The listing builds one solid part. Answer for the finished solid, in the listing's coordinates (mm). A direction names the side the tool comes from. Round coordinates to 2 decimals unless told otherwise and drop trailing zeros. Write each loop counter-clockwise with the first axis right and the second up, starting at its lowest first coordinate (ties: lowest second). Pieces come first, ordered by that corner, then holes. Notation, with made-up numbers: M -10,19 L 45,19 A12 cw 45,38 Z; hole C 81.5,7.25 d6. An arc over 180 degrees is marked long. Write each question's results on one line, items separated by ' | '.
from build123d import *

# Parameters (mm, degrees)
BOSS_EXTRUDE1_DEPTH     = 38.1
CUT_EXTRUDE1_DEPTH      = 35.56
CUT_EXTRUDE9_DEPTH      = 110.891333521
CUT_EXTRUDE9_DEPTH_BACK = 110.891333521
SKETCH20_R              = 2.54
BOSS_EXTRUDE2_DEPTH     = 0.635
SKETCH9_R               = 1.905
CUT_EXTRUDE4_DEPTH      = 3.175
BOSS_EXTRUDE3_DEPTH     = 0.635
SKETCH12_R              = 1.905
CUT_EXTRUDE5_DEPTH      = 0.635
SKETCH13_R              = 12.7
BOSS_EXTRUDE4_DEPTH     = 0.635
SKETCH14_R              = 12.7
CUT_EXTRUDE6_DEPTH      = 0.635
SKETCH15_R              = 12.7
CUT_EXTRUDE7_DEPTH      = 0.635
SKETCH16_R              = 12.7
CUT_EXTRUDE8_DEPTH      = 0.635
FILLET1_R               = 10.16
FILLET2_R               = 10.16


with BuildPart() as part:
    # Sketch3 → Boss-Extrude1 (new body)
    with BuildSketch(Plane.XY):
        Polygon((-22.959817584, 0), (22.959817584, 0), (46.332381312, 23.372563728), (46.332381312, 69.294099898), (23.55148121, 92.075), (-22.368153958, 92.075), (-45.740717686, 68.702436272), (-45.740717686, 22.780900102), align=None)
    extrude(amount=BOSS_EXTRUDE1_DEPTH)

    # Sketch4 → Cut-Extrude1 (cut)
    with BuildSketch(Plane.XY.offset(38.1)):
        Polygon((23.225329451, 91.2876), (-22.042002199, 91.2876), (-44.953317686, 68.376284513), (-44.953317686, 23.107051861), (-22.633665825, 0.7874), (22.633665825, 0.7874), (45.544981312, 23.698715487), (45.544981312, 68.967948139), align=None)
    extrude(amount=-CUT_EXTRUDE1_DEPTH, mode=Mode.SUBTRACT)

    # Sketch20 → Cut-Extrude9 (cut, two sides: drawn at the far end of the back side and taken through both)
    with BuildSketch(Plane.XY.offset(-CUT_EXTRUDE9_DEPTH_BACK)):
        with Locations((0, 65.0748)):
            Circle(SKETCH20_R)
        with Locations((19.05, 46.0248)):
            Circle(SKETCH20_R)
        with Locations((0, 26.9748)):
            Circle(SKETCH20_R)
        with Locations((-19.05, 46.0248)):
            Circle(SKETCH20_R)
    extrude(amount=CUT_EXTRUDE9_DEPTH + CUT_EXTRUDE9_DEPTH_BACK, mode=Mode.SUBTRACT)

    # Sketch8 → Boss-Extrude2 (add)
    with BuildSketch(Plane.XY.offset(38.1)):
        with BuildLine():
            Line((24.678794584, 77.195818088), (32.28681384, 83.33966737))
            Line((32.28681384, 83.33966737), (37.705421486, 77.921059725))
            Line((37.705421486, 77.921059725), (30.09740223, 71.777210443))
            ThreePointArc((30.09740223, 71.777210443), (24.639652924, 71.738068783), (24.678794584, 77.195818088))
        make_face()
    extrude(amount=-BOSS_EXTRUDE2_DEPTH)

    # Sketch9 → Cut-Extrude4 (cut)
    with BuildSketch(Plane.XY.offset(38.1)):
        with Locations((27.349235463, 74.447651321)):
            Circle(SKETCH9_R)
    extrude(amount=-CUT_EXTRUDE4_DEPTH, mode=Mode.SUBTRACT)

    # Sketch11 → Boss-Extrude3 (add)
    with BuildSketch(Plane.XY.offset(38.1)):
        with BuildLine():
            Line((-37.044344471, 14.084526887), (-30.129547258, 20.9993241))
            ThreePointArc((-30.129547258, 20.9993241), (-24.741393586, 20.9993241), (-24.741393586, 15.611170428))
            Line((-24.741393586, 15.611170428), (-31.656190799, 8.696373215))
            Line((-31.656190799, 8.696373215), (-37.044344471, 14.084526887))
        make_face()
    extrude(amount=-BOSS_EXTRUDE3_DEPTH)

    # Sketch12 → Cut-Extrude5 (cut)
    with BuildSketch(Plane.XY.offset(38.1)):
        with Locations((-27.435470422, 18.305247264)):
            Circle(SKETCH12_R)
    extrude(amount=-CUT_EXTRUDE5_DEPTH, mode=Mode.SUBTRACT)

    # Sketch13 → Boss-Extrude4 (add)
    with BuildSketch(Plane.XY.offset(2.54)):
        with Locations((0.284082314, 46.0502)):
            Circle(SKETCH13_R)
    extrude(amount=BOSS_EXTRUDE4_DEPTH)

    # Sketch14 → Cut-Extrude6 (cut)
    with BuildSketch(Plane(origin=(46.332381312, 0, 0), x_dir=(0, 0, -1), z_dir=(1, 0, 0))):
        with Locations((-19.05, 46.334163728)):
            Circle(SKETCH14_R)
    extrude(amount=-CUT_EXTRUDE6_DEPTH, mode=Mode.SUBTRACT)

    # Sketch15 → Cut-Extrude7 (cut)
    with BuildSketch(Plane.ZY.offset(45.740717686)):
        with Locations((19.05, 45.742500102)):
            Circle(SKETCH15_R)
    extrude(amount=-CUT_EXTRUDE7_DEPTH, mode=Mode.SUBTRACT)

    # Sketch16 → Cut-Extrude8 (cut)
    with BuildSketch(Plane.XZ):
        with Locations((0, 19.05)):
            Circle(SKETCH16_R)
    extrude(amount=-CUT_EXTRUDE8_DEPTH, mode=Mode.SUBTRACT)

    # Fillet1
    fillet1_edges = [part.edges().sort_by_distance(p)[0] for p in [
        (23.55148121, 92.075, 19.05),
        (46.332381312, 69.294099898, 19.05),
        (46.332381312, 23.372563728, 19.05),
        (22.959817584, 0, 19.05),
        (-22.959817584, 0, 19.05),
        (-45.740717686, 22.780900102, 19.05),
        (-45.740717686, 68.702436272, 19.05),
        (-22.368153958, 92.075, 19.05),
    ]]
    fillet(fillet1_edges, radius=FILLET1_R)

    # Fillet2
    fillet2_edges = [part.edges().sort_by_distance(p)[0] for p in [
        (23.225329451, 91.2876, 20.32),
        (45.544981312, 68.967948139, 20.32),
        (45.544981312, 23.698715487, 20.32),
        (22.633665825, 0.7874, 20.32),
        (-22.633665825, 0.7874, 20.32),
        (-44.953317686, 23.107051861, 20.32),
        (-44.953317686, 68.376284513, 20.32),
        (-22.042002199, 91.2876, 20.32),
    ]]
    fillet(fillet2_edges, radius=FILLET2_R)


solid = part.part
1) Section B-B (x = 0) is taken. Determine the outline of the cut face in (y, z) (3 decimals), then the cut area to 3 significant figures.
Return value:
outline: M 0,0 L 24.435,0 L 24.435,2.54 L 0.787,2.54 L 0.787,38.1 L 0,38.1 L 0,31.75 L 0.635,31.75 L 0.635,6.35 L 0,6.35 Z; M 29.515,0 L 62.535,0 L 62.535,2.54 L 58.747,2.54 L 58.747,3.175 L 33.353,3.175 L 33.353,2.54 L 29.515,2.54 Z; M 67.615,0 L 92.075,0 L 92.075,38.1 L 91.288,38.1 L 91.288,2.54 L 67.615,2.54 Z | area: 264 mm²
2) A tool of negligible diameter and unlimited length cuts with its end or side. For faces 1 (the face through (34.5, 80.013, 20.569)), 2 (the face through (46.332, 46, 6)), 3 (the face through (34.52, 11.56, 18.78)), 4 (the face through (-22.36, 1.58, 20.07)), 5 (the face through (-45.106, 46, 19)), from which of +Z, -Z, +X, -X, +Y, -Y can it reach the whole face along a straight path? Write none if from no direction.
Return value:
face 1: none | face 2: +Z, -Z, +X, +Y, -Y | face 3: +Z, -Z, +X, -Y | face 4: +Z | face 5: -X
3) Section C-C (y = 41.5) is taken. Determine the outline of the cut face in (x, z) (3 decimals).
Return value:
outline: M -45.741,0 L 46.332,0 L 46.332,7.306 L 45.697,7.306 L 45.697,30.794 L 46.332,30.794 L 46.332,38.1 L 45.545,38.1 L 45.545,2.54 L 12.141,2.54 L 12.141,3.175 L -11.573,3.175 L -11.573,2.54 L -44.953,2.54 L -44.953,38.1 L -45.741,38.1 L -45.741,31.02 L -45.106,31.02 L -45.106,7.08 L -45.741,7.08 Z
4) Find the intervals of material crossed by line 1 (Y direction, x = 0, z = 0.65) (3 decimals); line 2 (X direction, y = 64, z = 15); line 3 (X direction, y = 34, z = 21.5), in increasing order.
Return value:
line 1: 0 to 24.435, 29.515 to 62.535, 67.615 to 92.075 | line 2: -45.74 to -44.95, 45.54 to 46.33 | line 3: -45.11 to -44.95, 45.54 to 45.7
5) The mould has two halves that part along Z. Classify faces 6 (the face through (-2.75, 0.31, 6.65)), 7 (the face through (-2.469, 33.652, 2.853)), 8 (the face through (0, 0.635, 19)): +Z half, -Z half, draft (parallel to the pull), parting line (faces both ways), or undercut.
Return value:
face 6: undercut | face 7: draft | face 8: undercut
6) Each of these flat-tipped pins is pushed along its axis until it touches: pin 1 (20.5 mm diameter, centred on y = 45.74, z = 19.05, fed in from +X); pin 2 (4 mm diameter, centred on x = 0.5, z = 28, fed in from -Y) (3 decimals); pin 3 (20.5 mm diameter, centred on x = -2.5, y = 48, fed in from +Z) (3 decimals). Where does it stop, or does it pass through?
Return value:
pin 1: x = 45.7 | pin 2: y = 0.635 | pin 3: z = 3.175
